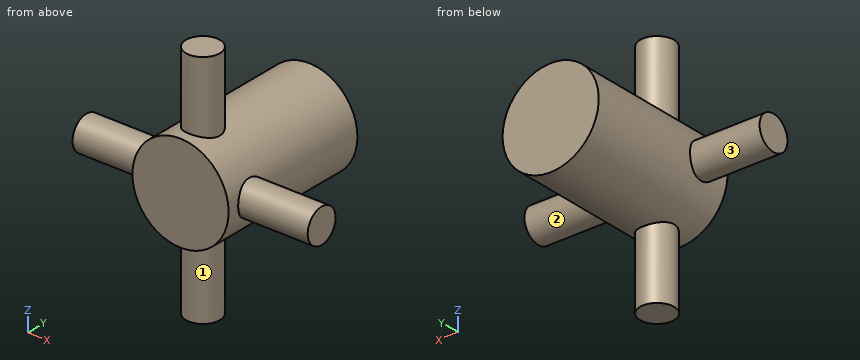
```python
from build123d import *

# Parameters (mm, degrees)
F0_R     = 31.1531
F1_DEPTH = 50.8
F2_R     = 10.9982
F4_DEPTH = 76.2
F3_R     = 10.9982
F5_DEPTH = 76.2


with BuildPart() as f1:
    # F0 (on Front) → F1 (new body, symmetric)
    with BuildSketch(Plane.XZ):
        Circle(F0_R)
    extrude(amount=F1_DEPTH, both=True)

    # F2 (on Right) → F4 (join, symmetric)
    with BuildSketch(Plane.YZ):
        with Locations((-32.224476, 0)):
            Circle(F2_R)
    extrude(amount=F4_DEPTH, both=True)

    # F3 (on Top) → F5 (join, symmetric)
    with BuildSketch(Plane.XY):
        with Locations((0, -33.121577)):
            Circle(F3_R)
    extrude(amount=F5_DEPTH, both=True)


solid = f1.part
```
Could you check a few things on this model? Use its own coordinates, in mm. Face numbers are marked on the shaded views. A direction names the side the tool comes from. Round coordinates to 2 decimals unless told otherwise and drop trailing zeros. Loops run counter-clockwise (first coordinate to the right, second up) from the corner with the lowest first, then second, coordinate; pieces in that order, holes last.
Q1. I want a section at B-B (x = 0). Write out the boundary of the cut face in (y, z), and give its area (3 significant figures).
Q2. On a 3-axis mill with a long thin cutter (end or side, diameter ignored), from which of +Z, -Z, +X, -X, +Y, -Y can I reach the whole of each face in a straight line? I mean the marked faces 1, 2 and 3. Say none if no direction works.
Q3. Please list where these lines run through material, in increasing order: L1, parallel to Z at x = -60.5, y = -33; L2, parallel to X at y = -17.5, z = -2; L3, parallel to X at y = -35, z = 50.
Q4. I want a section at C-C (y = 9). Write out the boundary of the cut face in (x, z).
Q5. I want a section at D-D (x = -51). Write out the boundary of the cut face in (y, z).
Q6. For P1, Ø2, axis at x = 34, y = -33, coming from the -Z side; P2, Ø6, axis at y = 27.5, z = -2, coming from the +X side; P3, Ø4, axis at y = -21, z = -11.5, coming from the +X side; P4, Ø4, axis at x = 23.5, z = -23.5, coming from the -Y side, each with a flat end and sliding along its axis, tell me the tip position at first contact or that it passes through.
Q7. I want a section at A-A (z = 0). Write out the boundary of the cut face in (x, y).
Answer below:
1. outline: (-50.8, -31.15) - (-44.12, -31.15) - (-44.12, -76.2) - (-22.12, -76.2) - (-22.12, -31.15) - (50.8, -31.15) - (50.8, 31.15) - (-22.12, 31.15) - (-22.12, 76.2) - (-44.12, 76.2) - (-44.12, 31.15) - (-50.8, 31.15) - close
1. area: 8,310 mm2
2. face 1: -Z
2. face 2: +X
2. face 3: -X
3. L1: z = -10.97 to 10.97
3. L2: x = -31.09 to 31.09
3. L3: x = -10.84 to 10.84
4. outline: circle Ø62.31 at (0, 0)
5. outline: circle Ø22 at (-32.22, 0)
6. P1: stops at z = -11
6. P2: stops at x = 31.15
6. P3: stops at x = 29.67
6. P4: passes through
7. outline: (-76.2, -43.22) - (-31.15, -43.22) - (-31.15, -50.8) - (31.15, -50.8) - (31.15, -43.22) - (76.2, -43.22) - (76.2, -21.23) - (31.15, -21.23) - (31.15, 50.8) - (-31.15, 50.8) - (-31.15, -21.23) - (-76.2, -21.23) - close
